Source: CAD feature listing. Evaluate the final solid. Frame: model axes, mm. A direction names the side the tool comes from. Round coordinates to 2 decimals unless told otherwise and drop trailing zeros. Order: outer loops, then holes, each group sorted by start corner. A loop starts at its lowest first (then second) coordinate and runs counter-clockwise, first axis right, second up. Notation, with made-up numbers: M 63.25,-35 L 121.25,-35 A21 ccw 121.25,-16 Z; hole C -29.75,32 d6. An arc over 180 degrees is marked long. Use one line per item in the form item = value. Start each with the question number.
Q1. Reachability of faces 1 (the flat face through (-15, 73, -109.613)), 2 (the cylindrical face through (59.1, 76, -105.9)) from +Z, -Z, +X, -X, +Y, -Y: full face, straight path, thin tool, end or side. Return the list, or none.
Q2. Section B-B (y = 24). Return the cut outline in (x, z).
Q3. Contact query for a flat-ended pin moving along its axis: pin 1 (4 mm diameter, centred on x = 18.5, z = -67, fed in from +Y). Output: stop coordinate, or through.
Q4. Material intervals for probe 1 along Z at (x, y) = (42, 71); probe 2 along X at (y, z) = (82, -81); probe 3 along Y at (x, z) = (-4, 23.5), sorted ascending.
Q5. Section C-C (x = -18.5). Return the cut outline in (y, z).
Q6. Section A-A (z = -7). Return the cut outline in (x, y).
Q7. Pull-direction query (Z, two-part tool) for faces 3 (the flat face through (-15, 0, -38)), 4 (the cylindrical face through (61.2, 75, -107.8)), 5 (the flat face through (-15, 74, -107.613)), 6 (the cylindrical face through (61.099, 75.036, 29.676)); classes: pulls with the +Z half, pulls with the -Z half, needs draft (parallel to the pull), parting line crosses it, or undercut.
from build123d import *

# Parameters (mm, degrees)
SKETCH1_W           = 154
SKETCH1_H           = 141
SKETCH1_W_2         = 150
SKETCH1_H_2         = 137
BOSS_EXTRUDE1_DEPTH = 148
SKETCH4_W           = 150
SKETCH4_H           = 137
BOSS_EXTRUDE2_DEPTH = 2
FILLET1_R           = 6
FILLET2_R           = 6
FILLET3_R           = 6
FILLET4_R           = 6
FILLET5_R           = 6
FILLET6_R           = 6
FILLET7_R           = 6
FILLET8_R           = 6


with BuildPart() as part:
    # Sketch1 → Boss-Extrude1 (new body)
    with BuildSketch(Plane(origin=(0, 0, 0), x_dir=(1, 0, 0), z_dir=(0, 1, 0))):
        with Locations((-14.096869638, 39.113007283)):
            Rectangle(SKETCH1_W, SKETCH1_H)
        with Locations((-14.096869638, 39.113007283)):
            Rectangle(SKETCH1_W_2, SKETCH1_H_2, mode=Mode.SUBTRACT)
    extrude(amount=BOSS_EXTRUDE1_DEPTH)

    # Sketch4 → Boss-Extrude2 (add)
    with BuildSketch(Plane.XZ):
        with Locations((-14.096869638, -39.113007283)):
            Rectangle(SKETCH4_W, SKETCH4_H)
    extrude(amount=-BOSS_EXTRUDE2_DEPTH)

    # Fillet1
    fillet1_edges = [part.edges().sort_by_distance(p)[0] for p in [
        (62.903130362, 74, 31.386992717),
    ]]
    fillet(fillet1_edges, radius=FILLET1_R)

    # Fillet2
    fillet2_edges = [part.edges().sort_by_distance(p)[0] for p in [
        (60.903130362, 75, 29.386992717),
    ]]
    fillet(fillet2_edges, radius=FILLET2_R)

    # Fillet3
    fillet3_edges = [part.edges().sort_by_distance(p)[0] for p in [
        (-89.096869638, 75, 29.386992717),
    ]]
    fillet(fillet3_edges, radius=FILLET3_R)

    # Fillet4
    fillet4_edges = [part.edges().sort_by_distance(p)[0] for p in [
        (-91.096869638, 74, 31.386992717),
    ]]
    fillet(fillet4_edges, radius=FILLET4_R)

    # Fillet5
    fillet5_edges = [part.edges().sort_by_distance(p)[0] for p in [
        (62.903130362, 74, -109.613007283),
    ]]
    fillet(fillet5_edges, radius=FILLET5_R)

    # Fillet6
    fillet6_edges = [part.edges().sort_by_distance(p)[0] for p in [
        (-91.096869638, 74, -109.613007283),
    ]]
    fillet(fillet6_edges, radius=FILLET6_R)

    # Fillet7
    fillet7_edges = [part.edges().sort_by_distance(p)[0] for p in [
        (-89.096869638, 75, -107.613007283),
    ]]
    fillet(fillet7_edges, radius=FILLET7_R)

    # Fillet8
    fillet8_edges = [part.edges().sort_by_distance(p)[0] for p in [
        (60.903130362, 75, -107.613007283),
    ]]
    fillet(fillet8_edges, radius=FILLET8_R)


solid = part.part
Results list:
q1.face_1 = -Z, +X, -X, +Y, -Y
q1.face_2 = +Y
q2.outline = M -91.1,-103.61 A6 ccw -85.1,-109.61 L 56.9,-109.61 A6 ccw 62.9,-103.61 L 62.9,25.39 A6 ccw 56.9,31.39 L -85.1,31.39 A6 ccw -91.1,25.39 Z; hole M -89.1,-101.61 A6 ccw -83.1,-107.61 L 54.9,-107.61 A6 ccw 60.9,-101.61 L 60.9,23.39 A6 ccw 54.9,29.39 L -83.1,29.39 A6 ccw -89.1,23.39 Z
q3.pin_1 = 2
q4.probe_1 = -109.61 to -107.61, 29.39 to 31.39
q4.probe_2 = -91.1 to -89.1, 60.9 to 62.9
q4.probe_3 = 0 to 2
q5.outline = M 0,-109.61 L 148,-109.61 L 148,-107.61 L 2,-107.61 L 2,29.39 L 148,29.39 L 148,31.39 L 0,31.39 Z
q6.outline = M -91.1,0 L 62.9,0 L 62.9,148 L 60.9,148 L 60.9,2 L -89.1,2 L -89.1,148 L -91.1,148 Z
q7.face_3 = needs draft
q7.face_4 = pulls with the -Z half
q7.face_5 = undercut
q7.face_6 = pulls with the +Z half
